```python
from build123d import *

# Parameters (mm, degrees)
F1_DEPTH = 8
F3_D     = 2.5
F3_DEPTH = 6
F3_TIP   = 0.7510757738
F5_D     = 2.5
F5_DEPTH = 6
F5_TIP   = 0.7510757738
F6_R     = 2
F7_W     = 3
F7_H     = 3
F8_DEPTH = 8.001
F9_R     = 1


with BuildPart() as f1:
    # F0 (on Front) → F1 (new body)
    with BuildSketch(Plane.XZ):
        with BuildLine():
            Line((-28.7, 0), (0, 0))
            Line((0, 0), (0, 28.7))
            Line((0, 28.7), (-3, 28.7))
            ThreePointArc((-3, 28.7), (-10.5273557235, 10.5273557235), (-28.7, 3))
            Line((-28.7, 3), (-28.7, 0))
        make_face()
    extrude(amount=F1_DEPTH)

    # F3
    with Locations(Plane.YZ):
        with Locations((-4, 14.35)):
            Hole(F3_D / 2, depth=F3_DEPTH)
            with Locations((0, 0, -(F3_DEPTH + F3_TIP / 2))):  # 118° drill point
                Cone(0, F3_D / 2, F3_TIP, mode=Mode.SUBTRACT)

    # F5
    with Locations(Plane(origin=(0, 0, 0), x_dir=(1, 0, 0), z_dir=(0, 0, -1))):
        with Locations((-14.35, 4)):
            Hole(F5_D / 2, depth=F5_DEPTH)
            with Locations((0, 0, -(F5_DEPTH + F5_TIP / 2))):  # 118° drill point
                Cone(0, F5_D / 2, F5_TIP, mode=Mode.SUBTRACT)

    # F6
    f6_edges = [f1.edges().sort_by_distance(p)[0] for p in [
        (-3, -4, 28.7),
        (-28.7, -4, 3),
    ]]
    fillet(f6_edges, radius=F6_R)

    # F7 (on face) → F8 (cut, through all)
    with BuildSketch(Plane.XZ.offset(8)):
        with Locations((-1.5, 1.5)):
            Rectangle(F7_W, F7_H)
    extrude(amount=-F8_DEPTH, mode=Mode.SUBTRACT)

    # F9
    f9_edges = [f1.edges().sort_by_distance(p)[0] for p in [
        (0, -4, 3),
        (-3, -4, 3),
        (-3, -4, 0),
    ]]
    fillet(f9_edges, radius=F9_R)


solid = f1.part
```
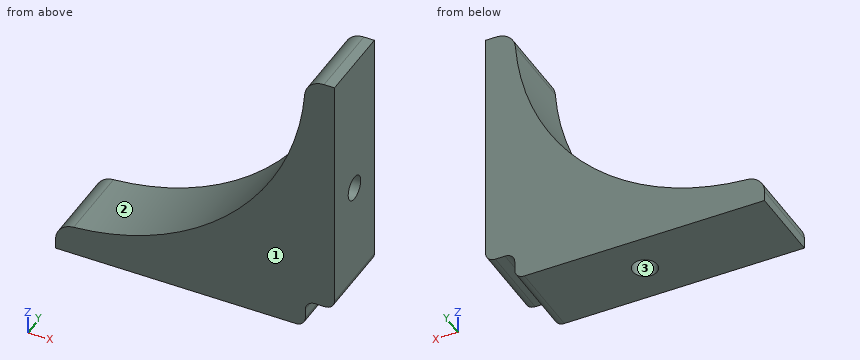
Verification items for the finished model (mm, model axes). Face numbers are marked on the shaded views. Give positions to 0.01 mm unless a question says otherwise; leave off trailing zeros. Loops run counter-clockwise (first coordinate to the right, second up) from the corner with the lowest first, then second, coordinate; pieces in that order, holes last.
1. Section check D-D, the plane x = -18.75. Enter the section's corners in (y, z), then the cut area to 3 significant figures.
2. Thickness scan on line 1 (Y direction, x = -3.7, z = 14.35); line 2 (X direction, y = -7.5, z = 1); line 3 (X direction, y = -1.5, z = 10.5). Record the ranges inside material, lowest first.
3. Go/stop test with flat-tipped pins: pin 1 Ø3 at (x, y) = (-3.5, -5) entering from +Z; pin 2 Ø4 at (y, z) = (-3, 9) entering from -X; pin 3 Ø2 at (x, y) = (-14.35, -4) entering from +Z. Record where each tip stops, or that it passes through.
4. Mould release check, pull along Y, two halves, no side actions. Record for the marked faces 1, 2 and 3: released by +Y, released by -Y, zero draft, split by the parting line, or undercut.
5. Section check A-A, the plane z = 4.75. Enter the section's corners in (x, y).
6. Section check C-C, the plane z = 12.5. Enter the section's corners in (x, y), then the cut area to 3 significant figures.
7. Section check B-B, the plane y = -6.75. Enter the section's corners in (x, z), then the cut area to 3 significant figures.
Geometry says:
1. outline: (-8, 0) - (0, 0) - (0, 5) - (-8, 5) - close
1. area: 40.0 mm2
2. line 1: y = -8 to -5.25, -2.75 to 0
2. line 2: x = -28.7 to -3
2. line 3: x = -10.55 to 0
3. pin 1: stops at z = 28.47
3. pin 2: stops at x = -14.93
3. pin 3: stops at z = 8.09
4. face 1: released by -Y
4. face 2: zero draft
4. face 3: undercut
5. outline: (-19.38, -8) - (0, -8) - (0, 0) - (-19.38, 0) - close; hole circle Ø2.5 at (-14.35, -4)
6. outline: (-8.75, -8) - (0, -8) - (0, 0) - (-8.75, 0) - close
6. area: 70.0 mm2
7. outline: (-28.7, 0) - (-4, 0) arc R1 ccw to (-3, 1) - (-3, 2) arc R1 cw to (-2, 3) - (-1, 3) arc R1 ccw to (0, 4) - (0, 28.7) - (-1.07, 28.7) arc R2 ccw to (-3.07, 26.84) arc R25.7 cw to (-26.84, 3.07) arc R2 ccw to (-28.7, 1.07) - close
7. area: 294 mm2
